Could you check a few things on this model? Use its own coordinates, in mm. A direction names the side the tool comes from. Give positions to 0.01 mm unless a question says otherwise; leave off trailing zeros. Loops run counter-clockwise (first coordinate to the right, second up) from the corner with the lowest first, then second, coordinate; pieces in that order, holes last. Notation, with made-up numbers: M 44.5,74 L 65.5,74 A18 ccw 65.5,78 Z; hole C 30.5,-32.75 d9. An arc over 180 degrees is marked long. Return JSON: item names as keys, results as strings. Group by question number.
1. For pin 1 (3 mm diameter, centred on x = 4, y = 3, fed in from -Z); pin 2 (3 mm diameter, centred on x = 8.5, z = 4.5, fed in from +Y), each with a flat end and sliding along its axis, tell me the tip position at first contact or that it passes through.
2. Please list where these lines run through material, in increasing order: line 1 (X direction, y = -3, z = 3.5); line 2 (Z direction, x = 5, y = -3); line 3 (X direction, y = -3.25, z = 4.5).
3. If we section it at A-A (y = 0): Write out the boundary of the cut face in (x, z), plus the area to 3 significant figures.
4. For faces 1 (the flat face through (8, 5, 3)), 2 (the cylindrical face through (10, 0, 6)), which set-ups out of +Z, -Z, +X, -X, +Y, -Y let a thin tool reach every point of the face, with its end or its side?
5. If we section it at D-D (x = 9.5): Write out the boundary of the cut face in (y, z), plus the area to 3 significant figures.
6. If we mould it in two halves opening along X, with no side actions, what happens to faces 3 (the cylindrical face through (1.007, 3.905, 0.867)), 4 (the flat face through (12, 0, 0)), 5 (the cylindrical face through (4.54, 4.88, 1.08)), 6 (the flat face through (0, 0, 0))? For each: +X half, -X half, draft (parallel to the pull), parting line (faces both ways), or undercut.
7. If we section it at C-C (x = 7): Write out the boundary of the cut face in (y, z).
```python
from build123d import *


with BuildPart() as part:
    # Sketch1 → Revolve1 (revolve)
    with BuildSketch(Plane(origin=(0, 0, 0), x_dir=(1, 0, 0), z_dir=(0, 1, 0))):
        with BuildLine():
            Line((0, 0), (0, 5))
            Line((0, 5), (0.5, 5))
            Line((0.5, 5), (0.5, 4))
            Line((0.5, 4), (1.5, 4))
            Line((1.5, 4), (1.5, 5))
            Line((1.5, 5), (7.5, 5))
            ThreePointArc((7.5, 5), (7.853553391, 5.146446609), (8, 5.5))
            Line((8, 5.5), (8, 6))
            Line((8, 6), (12, 6))
            Line((12, 6), (12, 0))
            Line((12, 0), (0, 0))
        make_face()
    revolve(axis=Axis((12, 0, 0), (-1, 0, 0)))


solid = part.part
```
Answer:
{
 "1": {"pin 1": "stops at z = -4.77", "pin 2": "stops at y = 5.2"},
 "2": {"line 1": "x = 0 to 0.5, 1.5 to 12", "line 2": "z = -4 to 4", "line 3": "x = 8 to 12"},
 "3": {"outline": "M 0,-5 L 0.5,-5 L 0.5,-4 L 1.5,-4 L 1.5,-5 L 7.5,-5 A0.5 cw 8,-5.5 L 8,-6 L 12,-6 L 12,6 L 8,6 L 8,5.5 A0.5 cw 7.5,5 L 1.5,5 L 1.5,4 L 0.5,4 L 0.5,5 L 0,5 Z", "area": "126 mm²"},
 "4": {"face 1": "-X", "face 2": "+X, -X"},
 "5": {"outline": "C 0,0 d12", "area": "113 mm²"},
 "6": {"face 3": "undercut", "face 4": "+X half", "face 5": "draft", "face 6": "-X half"},
 "7": {"outline": "C 0,0 d10"}
}
